Input: dimensioned drawing with shaded views. Units: mm. Origin: part minimum x, y, z. Give positions to 0.01 mm unless a question says otherwise; leave off trailing zeros. Write each loop counter-clockwise with the first axis right and the second up, starting at its lowest first coordinate (ties: lowest second). Pieces come first, ordered by that corner, then holes. Notation, with made-up numbers: (53.5, 60.25) -> (92.5, 60.25) arc R24 ccw to (92.5, 76.25) -> close; hole circle Ø9 at (63, 77). An arc over 180 degrees is marked (long way). Return JSON: item names as keys, results as strings. Group by question number.
Item 1: Section A-A, the plane x = 27.5. Return loops of the section in (y, z), then the cut area to 3 significant figures.
Item 2: Line query: line 1 (X direction, y = 2.5, z = 1.75); line 2 (Y direction, x = 29.5, z = 4); line 3 (X direction, y = 7.5, z = 5). Output: solid intervals per line, ascending. Write a range as [from, to].
Item 3: Pin query (flat end, axial travel): P1, Ø3, axis at x = 58, y = 4.5, coming from the +Z side; P2, Ø3, axis at x = 23.5, y = 4.5, coming from the -Z side; P3, Ø1, axis at x = 43, y = 6.5, coming from the -Z side. Return the tip coordinate at first contact, or that it passes through.
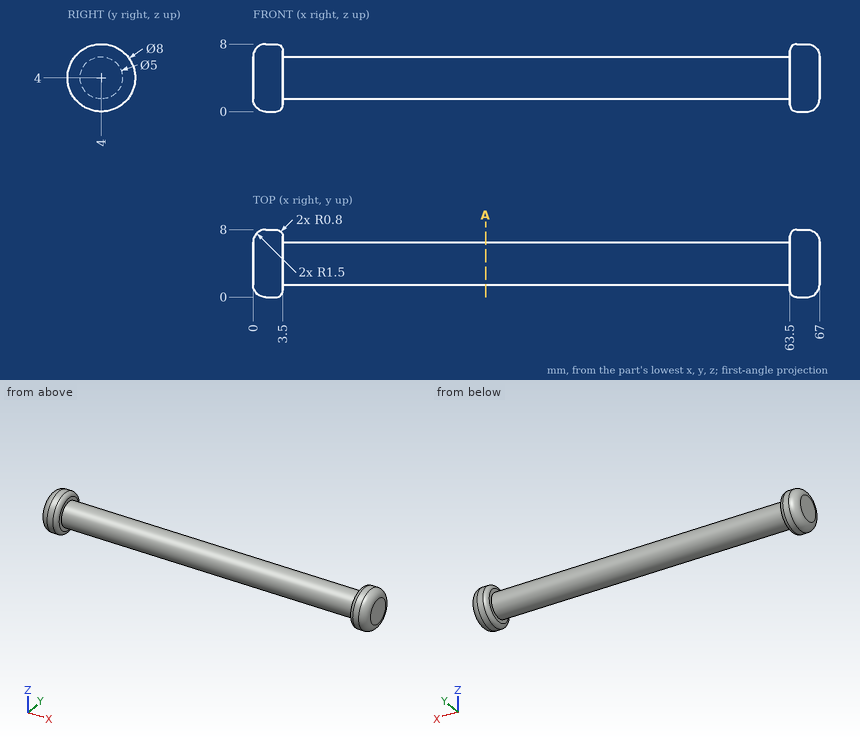
Answer below:
{
 "1": {"outline": "circle Ø5 at (4, 4)", "area": "19.6 mm2"},
 "2": {"line 1": "x = [0.01, 3.5], [63.5, 66.99]", "line 2": "y = [1.5, 6.5]", "line 3": "x = [0.53, 3.37], [63.63, 66.47]"},
 "3": {"P1": "stops at z = 6.5", "P2": "stops at z = 1.5", "P3": "stops at z = 2.5"}
}
